Here's how the part is built. I have some questions about the finished solid (model axes, mm). A direction names the side the tool comes from. Give positions to 0.01 mm unless a question says otherwise; leave off trailing zeros. Loops run counter-clockwise (first coordinate to the right, second up) from the corner with the lowest first, then second, coordinate; pieces in that order, holes last. Notation, with made-up numbers: M 89,57 L 96,57 A31 cw 96,93 Z; hole C 37,40 d8. An arc over 180 degrees is marked long. Answer as CSV lines item,"result". Start each with the question number.
Item 1: If we mould it in two halves opening along X, with no side actions, what happens to faces 4 (the flat face through (32.038, 0, -10)), 5 (the flat face through (0, -34.053, -10)), 6 (the cylindrical face through (-10.784, -2.233, -24.93)), 7 (the flat face through (-32.038, 0, -10))? For each: released by +X, released by -X, zero draft, split by the parting line, or undercut.
Item 2: I want a section at B-B on z = -25. List the corners of the cut face in (x, y) for me, plus the area to 3 significant figures.
Item 3: I want a section at A-A on y = 0. List the corners of the cut face in (x, z) for me, plus the area to 3 significant figures.
Item 4: If I drill on line 1 along Y through (x, z) = (-28, -6); line 2 along Z through (x, y) = (23.5, 80); line 3 along Z through (x, y) = (28.5, -28), over which ranges is the centre line in solid material (lowest first)? Write a range as from..to.
Item 5: I want a section at C-C on x = -18. List the corners of the cut face in (y, z) for me.
Item 6: I want a section at D-D on z = -8. List the corners of the cut face in (x, y) for me, plus the area to 3 significant figures.
Item 7: For faces 1 (the flat face through (-1, 9, 3)), 2 (the flat face through (0, 34.053, -10)), 3 (the cylindrical face through (22.93, -2.23, -24.93)), which set-ups out of +Z, -Z, +X, -X, +Y, -Y let a thin tool reach every point of the face, with its end or its side?
Item 8: Will these pins go through, and if not, where does the flat tip stop? P1, Ø6, axis at x = -9.5, z = -10.5, coming from the -Y side; P2, Ø3, axis at x = -4.5, y = 84.5, coming from the -Z side; P3, Ø3.5, axis at x = 49.5, z = 2, coming from the +Y side; P4, Ø8, axis at x = 50.5, z = -4.5, coming from the -Y side.
from build123d import *

# Parameters (mm, degrees)
SKETCH_1_W      = 140
SKETCH_1_H      = 100
EXTRUDE_1_DEPTH = 3
SKETCH_2_W      = 60
SKETCH_2_H      = 3
EXTRUDE_2_DEPTH = 50
SKETCH_3_W      = 64.075246498
SKETCH_3_H      = 68.106213914
EXTRUDE_3_DEPTH = 20
SKETCH_4_R      = 7.433229746
EXTRUDE_4_DEPTH = 10


with BuildPart() as part:
    # 草图1 → 凸台-拉伸1 (new body)
    with BuildSketch(Plane.XY):
        Rectangle(SKETCH_1_W, SKETCH_1_H)
    extrude(amount=EXTRUDE_1_DEPTH)

    # 草图2 → 凸台-拉伸2 (add)
    with BuildSketch(Plane(origin=(0, 50, 0), x_dir=(1, 0, 0), z_dir=(0, 1, 0))):
        with Locations((0, -1.5)):
            Rectangle(SKETCH_2_W, SKETCH_2_H)
    extrude(amount=EXTRUDE_2_DEPTH)

    # 草图3 → 凸台-拉伸3 (add)
    with BuildSketch(Plane(origin=(0, 0, 0), x_dir=(-1, 0, 0), z_dir=(0, 0, -1))):
        Rectangle(SKETCH_3_W, SKETCH_3_H)
    extrude(amount=EXTRUDE_3_DEPTH)

    # 草图4 → 凸台-拉伸4 (add)
    with BuildSketch(Plane(origin=(0, 0, -20), x_dir=(-1, 0, 0), z_dir=(0, 0, -1))):
        with Locations(Location((17.874179181, 0, 0), (0, 0, 180))):
            Circle(SKETCH_4_R)
        with Locations(Location((-15.837302871, 0, 0), (0, 0, 180))):
            Circle(SKETCH_4_R)
    extrude(amount=EXTRUDE_4_DEPTH)


solid = part.part
Result:
1,face 4,"released by +X"
1,face 5,"zero draft"
1,face 6,"undercut"
1,face 7,"released by -X"
2,outline,"C -17.87,0 d14.87; C 15.84,0 d14.87"
2,area,"347 mm^2"
3,outline,"M -70,0 L -32.04,0 L -32.04,-20 L -25.31,-20 L -25.31,-30 L -10.44,-30 L -10.44,-20 L 8.4,-20 L 8.4,-30 L 23.27,-30 L 23.27,-20 L 32.04,-20 L 32.04,0 L 70,0 L 70,3 L -70,3 Z"
3,area,"2,000 mm^2"
4,line 1,"-34.05..34.05"
4,line 2,"0..3"
4,line 3,"-20..3"
5,outline,"M -50,0 L -34.05,0 L -34.05,-20 L -7.43,-20 L -7.43,-30 L 7.43,-30 L 7.43,-20 L 34.05,-20 L 34.05,0 L 100,0 L 100,3 L -50,3 Z"
6,outline,"M -32.04,-34.05 L 32.04,-34.05 L 32.04,34.05 L -32.04,34.05 Z"
6,area,"4,360 mm^2"
7,face 1,"+Z, +X, -X, +Y, -Y"
7,face 2,"-Z, +X, -X, +Y"
7,face 3,"-Z"
8,P1,"y = -34.05"
8,P2,"z = 0"
8,P3,"y = 50"
8,P4,"through"
